Check sheet for the modelled part. Datum: model origin and axes. Units: mm. Face numbers are marked on the shaded views. A direction names the side the tool comes from. Give positions to 0.01 mm unless a question says otherwise; leave off trailing zeros. Loops run counter-clockwise (first coordinate to the right, second up) from the corner with the lowest first, then second, coordinate; pieces in that order, holes last. Notation, with made-up numbers: (80.25, 34.25) -> (100.25, 34.25) arc R8 ccw to (100.25, 47.25) -> close; hole circle Ø11 at (15, 9.25). An arc over 180 degrees is marked (long way). Write each question's results on one line, items separated by ' | '. Start each with the question number.
Item 1: Access from +Z, -Z, +X, -X, +Y, -Y to the whole of each face (thin tool, end or side, straight path). Record for the marked faces 1 and 2.
Item 2: Scan lines: line 1 along Z through (x, y) = (12.5, 3.5); line 2 along Y through (x, z) = (74, -34); line 3 along X through (y, z) = (9.5, -51.5). Record each from-to range of solid material in increasing order.
Item 3: Cross-section at B-B on z = -51.5. Enter the section's corners in (x, y), then the cut area to 3 significant figures.
Item 4: Cross-section at A-A on x = 47. Enter the section's corners in (y, z).
Item 5: Gauge pin test, flat ends, axial feed: pin 1 Ø12.5 at (y, z) = (6.5, -67.5) entering from +X; pin 2 Ø20.5 at (x, y) = (72.5, 18) entering from -Z; pin 3 Ø1 at (x, z) = (64.5, -69.5) entering from +Y. Record the tip position at first contact, or that the pin passes through.
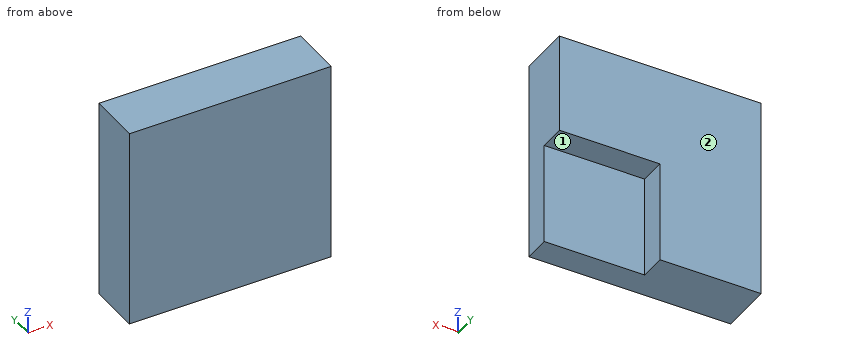
from build123d import *

# Parameters (mm, degrees)
F0_W     = 194.0150633454
F0_H     = 193.9053460956
F1_DEPTH = 25.4
F2_W     = 76.4794424176
F2_H     = 75.5990371108
F2_H_2   = 76.2040093541
F2_W_2   = 74.5813548565
F3_DEPTH = 25.4


with BuildPart() as f1:
    # F0 (on Front) → F1 (new body)
    with BuildSketch(Plane.XZ):
        with Locations((-0.3764815629, -0.8369870484)):
            Rectangle(F0_W, F0_H)
    extrude(amount=F1_DEPTH)

    # F2 (on face) → F3 (join)
    with BuildSketch(Plane(origin=(0, 0, 0), x_dir=(-1, 0, 0), z_dir=(0, 1, 0))):
        with Locations((38.2397212088, 37.7995185554)):
            Rectangle(F2_W, F2_H)
        with Locations((38.2397212088, -38.1020046771)):
            Rectangle(F2_W, F2_H_2)
        with Locations((-37.2906774282, 37.7995185554)):
            Rectangle(F2_W_2, F2_H)
        Polygon((97.3840132356, 0), (76.4794424176, 0), (76.4794424176, -76.2040093541), (0, -76.2040093541), (0, -97.7896600962), (97.3840132356, -97.7896600962), align=None)
        Polygon((76.4794424176, 75.5990371108), (76.4794424176, 0), (97.3840132356, 0), (97.3840132356, 96.1156859994), (-96.6310501099, 96.1156859994), (-96.6310501099, 0), (-74.5813548565, 0), (-74.5813548565, 75.5990371108), (0, 75.5990371108), align=None)
    extrude(amount=F3_DEPTH)


solid = f1.part
Answer sheet:
1) face 1: -Z, +X, +Y | face 2: +Z, -Z, +X, -X, +Y
2) line 1: z = 0 to 96.12 | line 2: y = -25.4 to 0 | line 3: x = -97.38 to 0
3) outline: (-97.38, -25.4) -> (96.63, -25.4) -> (96.63, 0) -> (0, 0) -> (0, 25.4) -> (-97.38, 25.4) -> close | area: 7,400 mm²
4) outline: (-25.4, -97.79) -> (0, -97.79) -> (0, 0) -> (25.4, 0) -> (25.4, 96.12) -> (-25.4, 96.12) -> close
5) pin 1: stops at x = 0 | pin 2: stops at z = 0 | pin 3: stops at y = 0
